Build history of the part. All positions in model axes, mm. A direction names the side the tool comes from. Give positions to 0.01 mm unless a question says otherwise; leave off trailing zeros. Write each loop counter-clockwise with the first axis right and the second up, starting at its lowest first coordinate (ties: lowest second). Pieces come first, ordered by that corner, then holes. Notation, with made-up numbers: M 8.25,22 L 43.25,22 A15 cw 43.25,40 Z; hole C 70,-16.5 d7. An arc over 180 degrees is marked long. One line per item, written item: value. Start each with the question number.
from build123d import *

# Parameters (mm, degrees)
SZKIC1_W                                             = 140
SZKIC1_H                                             = 350
DODANIE_WYCI_GNI_CIE1_DEPTH                          = 13
SZKIC2_W                                             = 46
SZKIC2_H                                             = 350
WYTNIJ_WYCI_GNI_CIE1_DEPTH                           = 1
OTW_R_GWINTOWANY_M5X0_81_D                           = 4.2
OTW_R_GWINTOWANY_M5X0_81_DEPTH                       = 35
OTW_R_GWINTOWANY_M5X0_81_TIP                         = 1.2618073
SZKIC12_W                                            = 48
SZKIC12_H                                            = 40
WYTNIJ_WYCI_GNI_CIE3_DEPTH                           = 1
POG_BIENIE_WALCOWE_POD_M5_WKR_T_DO_CZ_CI_D           = 5.5
POG_BIENIE_WALCOWE_POD_M5_WKR_T_DO_CZ_CI_CBORE_D     = 9
POG_BIENIE_WALCOWE_POD_M5_WKR_T_DO_CZ_CI_CBORE_DEPTH = 6
POG_BIENIE_WALCOWE_POD_M5_WKR_T_DO_C_2_D             = 5.5
POG_BIENIE_WALCOWE_POD_M5_WKR_T_DO_C_2_CBORE_D       = 9
POG_BIENIE_WALCOWE_POD_M5_WKR_T_DO_C_2_CBORE_DEPTH   = 5


with BuildPart() as part:
    # Szkic1 → Dodanie-wyciągnięcie1 (new body)
    with BuildSketch(Plane(origin=(0, 0, 0), x_dir=(1, 0, 0), z_dir=(0, 1, 0))):
        with Locations((70, 175)):
            Rectangle(SZKIC1_W, SZKIC1_H)
    extrude(amount=DODANIE_WYCI_GNI_CIE1_DEPTH)

    # Szkic2 → Wytnij-wyciągnięcie1 (cut)
    with BuildSketch(Plane.XZ):
        with Locations((23, -175)):
            Rectangle(SZKIC2_W, SZKIC2_H)
        with Locations((117, -175)):
            Rectangle(SZKIC2_W, SZKIC2_H)
    extrude(amount=-WYTNIJ_WYCI_GNI_CIE1_DEPTH, mode=Mode.SUBTRACT)

    # Otwór gwintowany M5x0.81
    with Locations(Plane(origin=(0, 0, -350), x_dir=(-1, 0, 0), z_dir=(0, 0, -1))):
        with Locations((-130, 7), (-105, 7), (-35, 7), (-10, 7)):
            Hole(OTW_R_GWINTOWANY_M5X0_81_D / 2, depth=OTW_R_GWINTOWANY_M5X0_81_DEPTH)
            with Locations((0, 0, -(OTW_R_GWINTOWANY_M5X0_81_DEPTH + OTW_R_GWINTOWANY_M5X0_81_TIP / 2))):  # 118° drill point
                Cone(0, OTW_R_GWINTOWANY_M5X0_81_D / 2, OTW_R_GWINTOWANY_M5X0_81_TIP, mode=Mode.SUBTRACT)

    # Szkic12 → Wytnij-wyciągnięcie3 (cut)
    with BuildSketch(Plane(origin=(0, 0, 0), x_dir=(-1, 0, 0), z_dir=(0, -1, 0))):
        with Locations((-70, 80)):
            Rectangle(SZKIC12_W, SZKIC12_H)
        with Locations((-70, 330)):
            Rectangle(SZKIC12_W, SZKIC12_H)
    extrude(amount=-WYTNIJ_WYCI_GNI_CIE3_DEPTH, mode=Mode.SUBTRACT)

    # Pog_bienie walcowe pod M5 Wkr_t do cz_ci (through all)
    with Locations(Plane(origin=(0, 13, 0), x_dir=(1, 0, 0), z_dir=(0, 1, 0))):
        with Locations((51, 344), (89, 344), (51, 324), (89, 324)):
            CounterBoreHole(POG_BIENIE_WALCOWE_POD_M5_WKR_T_DO_CZ_CI_D / 2, POG_BIENIE_WALCOWE_POD_M5_WKR_T_DO_CZ_CI_CBORE_D / 2, POG_BIENIE_WALCOWE_POD_M5_WKR_T_DO_CZ_CI_CBORE_DEPTH)

    # Pog_bienie walcowe pod M5 Wkr_t do c 2 (through all)
    with Locations(Plane(origin=(0, 13, 0), x_dir=(1, 0, 0), z_dir=(0, 1, 0))):
        with Locations((53, 85), (87, 85), (53, 75), (87, 75)):
            CounterBoreHole(POG_BIENIE_WALCOWE_POD_M5_WKR_T_DO_C_2_D / 2, POG_BIENIE_WALCOWE_POD_M5_WKR_T_DO_C_2_CBORE_D / 2, POG_BIENIE_WALCOWE_POD_M5_WKR_T_DO_C_2_CBORE_DEPTH)


solid = part.part
1) Tool access for faces 1 (the face through (70, 0, -206)), 2 (the face through (87, 8, -82)): list every direction of +Z, -Z, +X, -X, +Y, -Y with a clear straight run to the whole face (end or side of a thin tool).
2) Probe line 1 along X through (y, z) = (3.25, -75); line 2 along X through (y, z) = (9.4, -75); line 3 along Z through (x, y) = (88.5, 12). List the from-to ranges inside material, lowest first. Write a range as from..to.
3) Mould opens along Z. For faces 3 (the face through (0, 7, -173)), 4 (the face through (69, 6, 0)), 5 (the face through (85.4, 10, -321.3)) say: released by +Z, released by -Z, zero draft, split by the parting line, or undercut.
4) Band-saw the part on A-A (z = -262.5). List the corners of the cut face in (x, y).
5) Drop flat-ended pins along their axis: P1, Ø10, axis at x = 88, z = -84, coming from the +Y side; P2, Ø9, axis at x = 87, z = -85, coming from the -Y side; P3, Ø4.5, axis at x = 53, z = -85, coming from the -Y side; P4, Ø8, axis at x = 51, z = -344, coming from the +Y side. Give the stop position or say it passes through.
Model answer:
1. face 1: +Z, -Z, +X, -X, -Y
1. face 2: +Y
2. line 1: x = 0..50.25, 55.75..84.25, 89.75..140
2. line 2: x = 0..48.5, 57.5..82.5, 91.5..140
2. line 3: z = -350..-348.47, -339.53..-328.47, -319.53..-89.24, -80.76..-79.24, -70.76..0
3. face 3: zero draft
3. face 4: released by +Z
3. face 5: undercut
4. outline: M 0,1 L 46,1 L 46,0 L 94,0 L 94,1 L 140,1 L 140,13 L 0,13 Z
5. P1: stops at y = 13
5. P2: stops at y = 1
5. P3: passes through
5. P4: stops at y = 7
